Here's how the part is built. I have some questions about the finished solid (model axes, mm). A direction names the side the tool comes from. Coordinates: 2 decimals unless noted, no trailing zeros. Write each loop counter-clockwise with the first axis right and the second up, starting at its lowest first coordinate (ties: lowest second). Pieces come first, ordered by that corner, then holes. Notation, with made-up numbers: M -6,8 L 2,8 A17 cw 2,34 Z; hole C 51.5,23 d11. An arc over 180 degrees is marked long. Use a Markdown table: item, result.
Autodesk Inventor part; units mm, degrees
ref_plane "YZ Plane" through (0, 0, 0) normal (1, 0, 0) x (0, 1, 0)
ref_plane "XZ Plane" through (0, 0, 0) normal (0, 1, 0) x (-1, 0, 0)
ref_plane "XY Plane" through (0, 0, 0) normal (0, 0, 1) x (1, 0, 0)
sketch "Sketch1" plane through (0, 0, 0) normal (0, 0, 1) x (1, 0, 0)
  arc A0 (0, 6.3881) -> (0, -6.3881) centre (0, 0) ccw
  line L0 (-25.4, 7.9375) -> (-4.5511, -6.5496)
  line L1 (0, 7.9375) -> (0, -13.1033) construction
  line L2 (-25.4, 7.9375) -> (0, 7.9375)
  arc A1 (-4.5511, -6.5496) -> (0, -7.9756) centre (0, 0) ccw
  arc A2 (0, -6.3881) -> (0, 6.3881) centre (0, 0) ccw
  line L3 (25.4, 7.9375) -> (4.5511, -6.5496)
  line L4 (25.4, 7.9375) -> (0, 7.9375)
  arc A3 (0, -7.9756) -> (4.5511, -6.5496) centre (0, 0) ccw
  dimension "d0" = 12.7762
  dimension "d1" = 7.9375
  dimension "d2" = 25.4
  dimension "d3" = 1.5875
extrude "Plate1" add sketch "Sketch1" along normal blind 1.5875
sketch "Sketch2" plane through (25.4, 9.2075, -1.27) normal (0, 1, 0) x (-1, 0, 0)
  line L0 (50.8, 0) -> (0, 0)
  line L1 (0, 0) -> (0, -9.8425)
  line L2 (0, -9.8425) -> (50.8, -9.8425)
  line L3 (50.8, -9.8425) -> (50.8, 0)
edge flange "Flange1" height 12.7 angle 90 thickness 1.5875 bend radius 1.27 thickness toward (0, 1, 0) relief tear relief width 1.5875 relief depth 0.7937 edges at (-12.7, 7.9375, 0) wall of the first edge with corners at (-25.4, 9.2075, -1.27) (25.4, 9.2075, -1.27) (25.4, 9.2075, -11.1125) (-25.4, 9.2075, -11.1125)
bend "Bend1"
corner "Corner1"
sketch "Sketch3" plane through (-25.4, 10.795, -11.1125) normal (0, 1, 0) x (1, 0, 0)
  line L0 (0, -9.8425) -> (50.8, -9.8425)
  line L1 (50.8, 0) -> (50.8, -9.8425)
  line L2 (25.4, -6.2418) -> (25.4, -0.3175) construction
  circle A0 centre (25.4, -5.08) radius 2.0828
  dimension "d35" = 4.1656
  dimension "d36" = 4.7625
  dimension "d37" = 25.4
extrude "Cut1" cut sketch "Sketch3" against normal blind 1.5875
sketch "Sketch4" plane through (25.4, 7.9375, -12.3825) normal (0, 0, -1) x (-1, 0, 0)
  line L0 (50.8, 0) -> (0, 0)
  line L1 (0, 0) -> (0, -16.2306)
  line L2 (0, -16.2306) -> (50.8, -16.2306)
  line L3 (50.8, -16.2306) -> (50.8, 0)
edge flange "Flange2" height 19.0881 angle 90 thickness 1.5875 bend radius 1.27 thickness toward (0, 0, -1) relief tear relief width 1.5875 relief depth 0.7937 edges at (0, 9.2075, -11.1125) wall of the first edge with corners at (-25.4, 7.9375, -12.3825) (25.4, 7.9375, -12.3825) (25.4, -8.2931, -12.3825) (-25.4, -8.2931, -12.3825)
bend "Bend2"
corner "Corner2"
sketch "Sketch5" plane through (25.4, -8.2931, -13.97) normal (0, 0, -1) x (-1, 0, 0)
  line L0 (50.8, 16.2306) -> (0, 16.2306)
  line L1 (0, 0) -> (0, 16.2306)
  line L2 (50.8, 0) -> (0, 0)
  line L3 (50.8, 16.2306) -> (50.8, 0)
  circle A0 centre (25.4, 8.2931) radius 6.3881
  line L4 (50.8, 16.2306) -> (29.9511, 1.7435)
  line L5 (0, 16.2306) -> (50.8, 16.2306)
  line L6 (20.8489, 1.7435) -> (0, 16.2306)
  arc A1 (20.8489, 1.7435) -> (29.9511, 1.7435) centre (25.4, 8.2931) ccw
extrude "Cut2" cut sketch "Sketch5" against normal blind 1.5875 contours L3 L2 L1 L6 A1 L4 | A0
equation "\"d37\" = d2"
equation "\"d18\" = Thickness"
equation "\"d49\" = Thickness"
equation "\"d5\" = BendReliefWidth"
equation "\"d6\" = BendReliefDepth"
equation "\"d7\" = MinimumRemnant"
equation "\"d8\" = BendRadius"
equation "\"d12\" = CornerReliefSize"
equation "\"d13\" = GapSize"
equation "\"d14\" = JacobiRadiusSize"
equation "\"d39\" = BendReliefWidth"
equation "\"d40\" = BendReliefDepth"
equation "\"d41\" = MinimumRemnant"
equation "\"d42\" = BendRadius"
equation "\"d46\" = CornerReliefSize"
equation "\"d47\" = GapSize"
equation "\"d48\" = JacobiRadiusSize"
equation "\"BendRadius\" = Thickness"
equation "\"BendReliefWidth\" = Thickness"
equation "\"BendReliefDepth\" = 0.5 * Thickness"
equation "\"CornerReliefSize\" = 4 * Thickness"
equation "\"MinimumRemnant\" = 2 * Thickness"
equation "\"TransitionRadius\" = BendRadius"
equation "\"JacobiRadiusSize\" = BendRadius"
equation "\"GapSize\" = Thickness"
equation "\"d4\" = BendRadius"
properties part number "Pipe to Gas Spring Connector (9417K91)" material "Aluminum"
1. I need wall thicknesses on probe 1 along Z at (x, y) = (-5, 7.75); probe 2 along Y at (x, z) = (-13.5, -4) (1 decimal); probe 3 along Z at (x, y) = (0, 10.05). Which ranges of each line are inside material? Lowest first, please.
Answers follow:
| item | result |
|---|---|
| probe 1 | z = -13.97 to -12.38, 0 to 1.59 |
| probe 2 | y = 9.2 to 10.8 |
| probe 3 | z = -13.04 to -8.12, -3.95 to 0.65 |
2. We'd pull the mould along Z, two halves only. Please class faces 1 (the face through (-2.35, -7.62, 0.78)), 2 (the face through (0.356, 9.936, -13.155)), 3 (the face through (0.356, 8.845, -0.382)): +Z half, -Z half, draft (parallel to the pull), parting line (faces both ways), or undercut.
Answers follow:
| item | result |
|---|---|
| face 1 | draft |
| face 2 | -Z half |
| face 3 | undercut |
3. Which directions (+Z, -Z, +X, -X, +Y, -Y) give clear straight access to the entire face, cutting with the end or side of a thin tool? Please do faces 4 (the face through (-15.121, 0.795, -13.187)), 5 (the face through (0.4, 9.208, -8.3)).
Answers follow:
| item | result |
|---|---|
| face 4 | +Z, -Z, -X, -Y |
| face 5 | +X, -X, -Y |
4. Suppose I cut it at D-D on y = 8.75. Write out the boundary of the cut face in (x, z).
Answers follow:
| item | result |
|---|---|
| outline | M -25.4,-13.85 L 25.4,-13.85 L 25.4,-12.09 L -25.4,-12.09 Z; M -25.4,-0.29 L 25.4,-0.29 L 25.4,1.47 L -25.4,1.47 Z |
5. Suppose I cut it at C-C on x = 3.5. Write out the boundary of the cut face in (y, z) (1 decimal).
Answers follow:
| item | result |
|---|---|
| outline | M -7.2,-14 L -5.3,-14 L -5.3,-12.4 L -7.2,-12.4 Z; M -7.2,0 L -5.3,0 L -5.3,1.6 L -7.2,1.6 Z; M 5.3,-14 L 7.9,-14 A2.9 ccw 10.8,-11.1 L 10.8,-1.3 A2.9 ccw 7.9,1.6 L 5.3,1.6 L 5.3,0 L 7.9,0 A1.3 cw 9.2,-1.3 L 9.2,-11.1 A1.3 cw 7.9,-12.4 L 5.3,-12.4 Z |
6. Suppose I cut it at A-A on y = 1.5. Write out the boundary of the cut face in (x, z), and give its area (3 significant figures).
Answers follow:
| item | result |
|---|---|
| outline | M -16.14,-13.97 L -6.21,-13.97 L -6.21,-12.38 L -16.14,-12.38 Z; M -16.14,0 L -6.21,0 L -6.21,1.59 L -16.14,1.59 Z; M 6.21,-13.97 L 16.14,-13.97 L 16.14,-12.38 L 6.21,-12.38 Z; M 6.21,0 L 16.14,0 L 16.14,1.59 L 6.21,1.59 Z |
| area | 63.0 mm2 |
7. Will these pins go through, and if not, where does the flat tip stop? pin 1 Ø6 at (y, z) = (0.5, -11.5) entering from +X; pin 2 Ø8 at (x, z) = (-4, -6) entering from -Y.
Answers follow:
| item | result |
|---|---|
| pin 1 | stops at x = 18.82 |
| pin 2 | stops at y = 9.21 |
8. Suppose I cut it at B-B on z = -5.5. Write out the boundary of the cut face in (x, y) (1 decimal).
Answers follow:
| item | result |
|---|---|
| outline | M -25.4,9.2 L -2,9.2 L -2,10.8 L -25.4,10.8 Z; M 2,9.2 L 25.4,9.2 L 25.4,10.8 L 2,10.8 Z |
